Source: CAD feature listing. Evaluate the final solid. Frame: model axes, mm. A direction names the side the tool comes from. Coordinates: 2 decimals unless noted, no trailing zeros. Loops run counter-clockwise (first coordinate to the right, second up) from the corner with the lowest first, then second, coordinate; pieces in that order, holes last. Notation, with made-up numbers: (34.25, -36) - (39.25, -36) arc R17 cw to (39.25, -23) - close; hole circle Ø8 at (59, 74.5). An arc over 180 degrees is marked (long way). Use CSV: the item, a comma, the result in double quotes. Start each with the question number.
```python
from build123d import *

# Parameters (mm, degrees)
SKETCH1_R                    = 9.525
BOSS_EXTRUDE1_DEPTH          = 5.715
BOSS_EXTRUDE2_DEPTH          = 6.35
SKETCH3_R                    = 7.9375
BOSS_EXTRUDE3_DEPTH          = 1.058333333
SKETCH4_R                    = 7.6835
BOSS_EXTRUDE4_DEPTH          = 1.058333333
F_1_4_18_NPSM_TAPPED_HOLE2_D = 11.8872
SKETCH11_R                   = 10.998522628
SKETCH11_R_2                 = 9.525
CUT_EXTRUDE1_DEPTH           = 21.317795019


with BuildPart() as part:
    # Sketch1 → Boss-Extrude1 (new body)
    with BuildSketch(Plane(origin=(0, 0, 0), x_dir=(1, 0, 0), z_dir=(0, 1, 0))):
        with Locations(Location((0, 0, 0), (0, 0, 270))):
            Circle(SKETCH1_R)
    extrude(amount=BOSS_EXTRUDE1_DEPTH)

    # Sketch2 → Boss-Extrude2 (add)
    with BuildSketch(Plane.XZ):
        Polygon((0, -10.998522628), (9.525, -5.499261314), (9.525, 5.499261314), (0, 10.998522628), (-9.525, 5.499261314), (-9.525, -5.499261314), align=None)
    extrude(amount=BOSS_EXTRUDE2_DEPTH)

    # Sketch3 → Boss-Extrude3 (add)
    with BuildSketch(Plane.XZ.offset(6.35)):
        with Locations(Location((0, 0, 0), (0, 0, 270))):
            Circle(SKETCH3_R)
    extrude(amount=BOSS_EXTRUDE3_DEPTH)

    # Sketch4 → Boss-Extrude4 (add)
    with BuildSketch(Plane.XZ.offset(7.408333333)):
        with Locations(Location((0, 0, 0), (0, 0, 270))):
            Circle(SKETCH4_R)
    extrude(amount=BOSS_EXTRUDE4_DEPTH)

    # 1/4-18 NPSM Tapped Hole2 (through all)
    with Locations(Plane(origin=(0, 5.715, 0), x_dir=(1, 0, 0), z_dir=(0, 1, 0))):
        with Locations((0, 0)):
            Hole(F_1_4_18_NPSM_TAPPED_HOLE2_D / 2)

    # Sketch11 → Cut-Extrude1 (cut, through all)
    with BuildSketch(Plane(origin=(0, 5.715, 0), x_dir=(1, 0, 0), z_dir=(0, 1, 0))):
        Circle(SKETCH11_R)
        with Locations(Location((0, 0, 0), (0, 0, 90))):
            Circle(SKETCH11_R_2, mode=Mode.SUBTRACT)
    extrude(amount=-CUT_EXTRUDE1_DEPTH, mode=Mode.SUBTRACT)


solid = part.part
```
(1) Section D-D on z = -7.25. Output: boundary loops of the cut face in (x, y) (3 decimals), plus the area to 3 significant figures.
(2) Draft query along Z for faces 3 (the cylindrical face through (-5.669, -1.475, -1.785)), 4 (the flat face through (-2, -6.35, 8)), 5 (the cylindrical face through (5.796, -0.233, 7.559)). Return one class per face: released by +Z, released by -Z, zero draft, split by the parting line, or undercut.
(3) Ray query, line 1 (Y direction, x = 6.75, z = -5.5) (3 decimals); line 2 (Z direction, x = 1.75, y = 3); line 3 (X direction, y = -5, z = 2). Return the intervals inside material, ascending. Write a range as [from, to].
(4) Reachability of faces 1 (the flat face through (-5, -8.467, -4)), 2 (the cylindrical face through (-7.5, -7.93, 1.67)) from +Z, -Z, +X, -X, +Y, -Y: full face, straight path, thin tool, end or side. Return the list, or none.
(5) Pin query (flat end, axial travel): pin 1 Ø2 at (x, y) = (2.5, 3) entering from -Z; pin 2 Ø1.5 at (y, z) = (-7, 1) entering from -X; pin 3 Ø4 at (x, y) = (4.5, -4) entering from -Z. Return the tip coordinate at first contact, or that it passes through.
(6) Section C-C on y = 2. Output: boundary loops of the cut face in (x, z) (3 decimals).
Solution:
1,outline,"(-6.178, -6.35) - (-3.231, -6.35) - (-3.231, -7.408) - (-2.544, -7.408) - (-2.544, -8.467) - (2.544, -8.467) - (2.544, -7.408) - (3.231, -7.408) - (3.231, -6.35) - (6.178, -6.35) - (6.178, 5.715) - (-6.178, 5.715) - close"
1,area,"161 mm²"
2,face 3,"undercut"
2,face 4,"zero draft"
2,face 5,"split by the parting line"
3,line 1,"y = [-6.35, 5.715]"
3,line 2,"z = [-9.36, -5.68], [5.68, 9.36]"
3,line 3,"x = [-9.31, -5.6], [5.6, 9.31]"
4,face 1,"+Z, -Z, +X, -X, -Y"
4,face 2,"-Y"
5,pin 1,"stops at z = -9.41"
5,pin 2,"stops at x = -9.5"
5,pin 3,"stops at z = -9.19"
6,outline,"circle Ø19.05 at (0, 0); hole circle Ø11.887 at (0, 0)"
